Here's how the part is built. I have some questions about the finished solid (model axes, mm). Face numbers are marked on the shaded views. A direction names the side the tool comes from. Round coordinates to 2 decimals unless told otherwise and drop trailing zeros. Answer as CSV lines item,"result".
```python
from build123d import *

# Parameters (mm, degrees)
SKIZZE1_R                            = 70
AUFSATZ_LINEAR_AUSTRAGEN1_DEPTH      = 4
SCHNITT_LINEAR_AUSTRAGEN1_REACH      = 6
SKIZZE2_R                            = 2.5
SKIZZE2_R_2                          = 1.5
AUFSATZ_LINEAR_AUSTRAGEN2_DEPTH      = 6
AUFSATZ_LINEAR_AUSTRAGEN2_DEPTH_BACK = 4
SKIZZE4_R                            = 1.5
SKIZZE4_R_2                          = 1.410083192
SCHNITT_LINEAR_AUSTRAGEN2_DEPTH      = 5
FASE1_SIZE                           = 0.5
SCHNITT_LINEAR_AUSTRAGEN3_REACH      = 12
SKIZZE5_R                            = 1.35
SKIZZE6_R                            = 1.6
SCHNITT_LINEAR_AUSTRAGEN4_DEPTH      = 4


with BuildPart() as part:
    # Skizze1 → Aufsatz-Linear austragen1 (new body)
    with BuildSketch(Plane(origin=(0, 0, 0), x_dir=(1, 0, 0), z_dir=(0, 1, 0))):
        Circle(SKIZZE1_R)
    extrude(amount=AUFSATZ_LINEAR_AUSTRAGEN1_DEPTH)

    # Skizze3 → Schnitt-Linear austragen1 (cut, up to next)
    with BuildSketch(Plane.XZ, mode=Mode.PRIVATE) as schnitt_linear_austragen1_sk1:
        with BuildLine():
            Line((6, -10), (0, -10))
            ThreePointArc((0, -10), (-10, 0), (0, 10))
            Line((0, 10), (6, 10))
            ThreePointArc((6, 10), (16, 0), (6, -10))
        make_face()
    schnitt_linear_austragen1_tool1 = extrude(schnitt_linear_austragen1_sk1.sketch, amount=-SCHNITT_LINEAR_AUSTRAGEN1_REACH, mode=Mode.PRIVATE) & part.part
    add(schnitt_linear_austragen1_tool1.solids().sort_by_distance((3, 0, 0))[0], mode=Mode.SUBTRACT)

    # Skizze2 → Aufsatz-Linear austragen2 (add, two sides)
    with BuildSketch(Plane(origin=(0, 4, 0), x_dir=(1, 0, 0), z_dir=(0, 1, 0))) as aufsatz_linear_austragen2_sk:
        with Locations((-47.533988615, 40.571841958)):
            Circle(SKIZZE2_R)
        with Locations((-5.293377745, 17.030303573)):
            Circle(SKIZZE2_R)
        with Locations((-47.533988615, -33.027520141)):
            Circle(SKIZZE2_R)
        with Locations((-32.533187453, 16.85488412)):
            Circle(SKIZZE2_R)
        with Locations((-32.533187453, 16.85488412)):
            Circle(SKIZZE2_R_2, mode=Mode.SUBTRACT)
        with Locations((-0.280707317, 46.779952313)):
            Circle(SKIZZE2_R)
        with Locations((-0.280707317, 46.779952313)):
            Circle(SKIZZE2_R_2, mode=Mode.SUBTRACT)
        with Locations((23.260650032, 28.271453094)):
            Circle(SKIZZE2_R)
        with Locations((23.260650032, 28.271453094)):
            Circle(SKIZZE2_R_2, mode=Mode.SUBTRACT)
        with Locations((45.260650032, 28.271453094)):
            Circle(SKIZZE2_R)
        with Locations((45.260650032, 28.271453094)):
            Circle(SKIZZE2_R_2, mode=Mode.SUBTRACT)
        with Locations((45.260650032, -28.428546906)):
            Circle(SKIZZE2_R)
        with Locations((45.260650032, -28.428546906)):
            Circle(SKIZZE2_R_2, mode=Mode.SUBTRACT)
        with Locations((23.260650032, -28.428546906)):
            Circle(SKIZZE2_R)
        with Locations((23.260650032, -28.428546906)):
            Circle(SKIZZE2_R_2, mode=Mode.SUBTRACT)
        with Locations((-0.152992521, -33.940171336)):
            Circle(SKIZZE2_R)
        with Locations((-0.152992521, -33.940171336)):
            Circle(SKIZZE2_R_2, mode=Mode.SUBTRACT)
    extrude(amount=AUFSATZ_LINEAR_AUSTRAGEN2_DEPTH)
    extrude(aufsatz_linear_austragen2_sk.sketch, amount=-AUFSATZ_LINEAR_AUSTRAGEN2_DEPTH_BACK)

    # Skizze4 → Schnitt-Linear austragen2 (cut, through all)
    with BuildSketch(Plane(origin=(0, 4, 0), x_dir=(1, 0, 0), z_dir=(0, 1, 0))):
        with Locations((-32.533187453, 16.85488412)):
            Circle(SKIZZE4_R)
        with Locations((23.260650032, 28.271453094)):
            Circle(SKIZZE4_R)
        with Locations((45.260650032, 28.271453094)):
            Circle(SKIZZE4_R)
        with Locations((45.260650032, -28.428546906)):
            Circle(SKIZZE4_R)
        with Locations((23.260650032, -28.428546906)):
            Circle(SKIZZE4_R)
        with Locations((-0.152992521, -33.940171336)):
            Circle(SKIZZE4_R)
        with Locations((-0.280707317, 46.779952313)):
            Circle(SKIZZE4_R_2)
    extrude(amount=-SCHNITT_LINEAR_AUSTRAGEN2_DEPTH, mode=Mode.SUBTRACT)

    # Fase1
    fase1_edges = [part.edges().sort_by_distance(p)[0] for p in [
        (-70, 0, 0),
    ]]
    chamfer(fase1_edges, length=FASE1_SIZE)

    # Skizze5 → Schnitt-Linear austragen3 (cut, up to next)
    with BuildSketch(Plane.XZ, mode=Mode.PRIVATE) as schnitt_linear_austragen3_sk1:
        with Locations((-55, 0)):
            Circle(SKIZZE5_R)
    schnitt_linear_austragen3_tool1 = extrude(schnitt_linear_austragen3_sk1.sketch, amount=-SCHNITT_LINEAR_AUSTRAGEN3_REACH, mode=Mode.PRIVATE) & part.part
    add(schnitt_linear_austragen3_tool1.solids().sort_by_distance((-55, 0, 0))[0], mode=Mode.SUBTRACT)
    # Skizze5 → Schnitt-Linear austragen3 (cut, up to next)
    with BuildSketch(Plane.XZ, mode=Mode.PRIVATE) as schnitt_linear_austragen3_sk2:
        with Locations((55, 0)):
            Circle(SKIZZE5_R)
    schnitt_linear_austragen3_tool2 = extrude(schnitt_linear_austragen3_sk2.sketch, amount=-SCHNITT_LINEAR_AUSTRAGEN3_REACH, mode=Mode.PRIVATE) & part.part
    add(schnitt_linear_austragen3_tool2.solids().sort_by_distance((55, 0, 0))[0], mode=Mode.SUBTRACT)
    # Skizze5 → Schnitt-Linear austragen3 (cut, up to next)
    with BuildSketch(Plane.XZ, mode=Mode.PRIVATE) as schnitt_linear_austragen3_sk3:
        with Locations((0, -55)):
            Circle(SKIZZE5_R)
    schnitt_linear_austragen3_tool3 = extrude(schnitt_linear_austragen3_sk3.sketch, amount=-SCHNITT_LINEAR_AUSTRAGEN3_REACH, mode=Mode.PRIVATE) & part.part
    add(schnitt_linear_austragen3_tool3.solids().sort_by_distance((0, 0, -55))[0], mode=Mode.SUBTRACT)
    # Skizze5 → Schnitt-Linear austragen3 (cut, up to next)
    with BuildSketch(Plane.XZ, mode=Mode.PRIVATE) as schnitt_linear_austragen3_sk4:
        with Locations((0, 55)):
            Circle(SKIZZE5_R)
    schnitt_linear_austragen3_tool4 = extrude(schnitt_linear_austragen3_sk4.sketch, amount=-SCHNITT_LINEAR_AUSTRAGEN3_REACH, mode=Mode.PRIVATE) & part.part
    add(schnitt_linear_austragen3_tool4.solids().sort_by_distance((0, 0, 55))[0], mode=Mode.SUBTRACT)

    # Skizze6 → Schnitt-Linear austragen4 (cut)
    with BuildSketch(Plane(origin=(0, 0, 0), x_dir=(-1, 0, 0), z_dir=(0, -1, 0))):
        with Locations((-10.644187298, 11.605236936)):
            Circle(SKIZZE6_R)
        with Locations((-10.644187298, -11.605236936)):
            Circle(SKIZZE6_R)
    extrude(amount=-SCHNITT_LINEAR_AUSTRAGEN4_DEPTH, mode=Mode.SUBTRACT)


solid = part.part
```
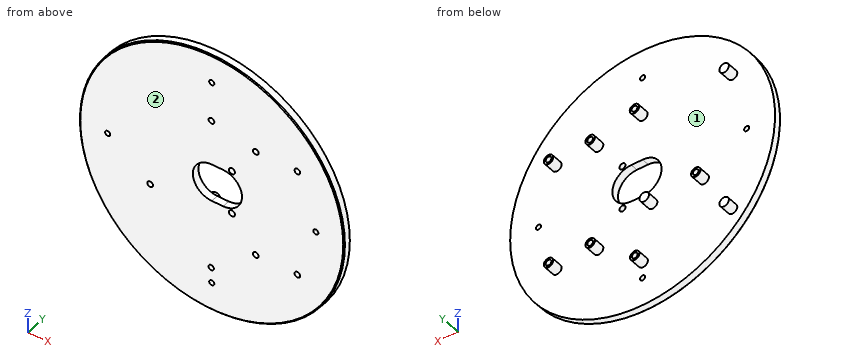
1. I want a section at A-A, the plane y = 7.25. Count the separate pieces of the cut face and the enclosed holes in it, and give its area (3 significant figures).
Evaluation:
separate pieces,"10"
enclosed holes,"7"
area,"147 mm²"
2. For P1, Ø5, axis at x = 10.64, z = 11.61, coming from the -Y side; P2, Ø3.5, axis at x = 0, z = 55, coming from the +Y side; P3, Ø1, axis at x = 1.5, y = 9, coming from the +Z side; P4, Ø4, axis at x = -15, y = 5, coming from the -Z side, each with a flat end and sliding along its axis, tell me the tip position at first contact or that it passes through.
Evaluation:
P1,"stops at y = 0"
P2,"stops at y = 4"
P3,"stops at z = 36.16"
P4,"stops at z = -68.73"
3. Which directions (+Z, -Z, +X, -X, +Y, -Y) give clear straight access to the entire face, cutting with the end or side of a thin tool? Please do the marked faces 1 and 2.
Evaluation:
face 1,"+Y"
face 2,"+Z, -Z, +X, -X, -Y"
4. If I drill on line 1 (Y direction, x = -31.5, z = 17.5); line 2 (Z direction, x = -32.5, y = 5.5); line 3 (X direction, y = 2.25, z = -56), over which ranges is the centre line in solid material (lowest first)? Write a range as [from, to].
Evaluation:
line 1,"y = [0, 4]"
line 2,"z = [-19.35, -18.35], [-15.36, -14.36]"
line 3,"x = [-42, -0.91], [0.91, 42]"
